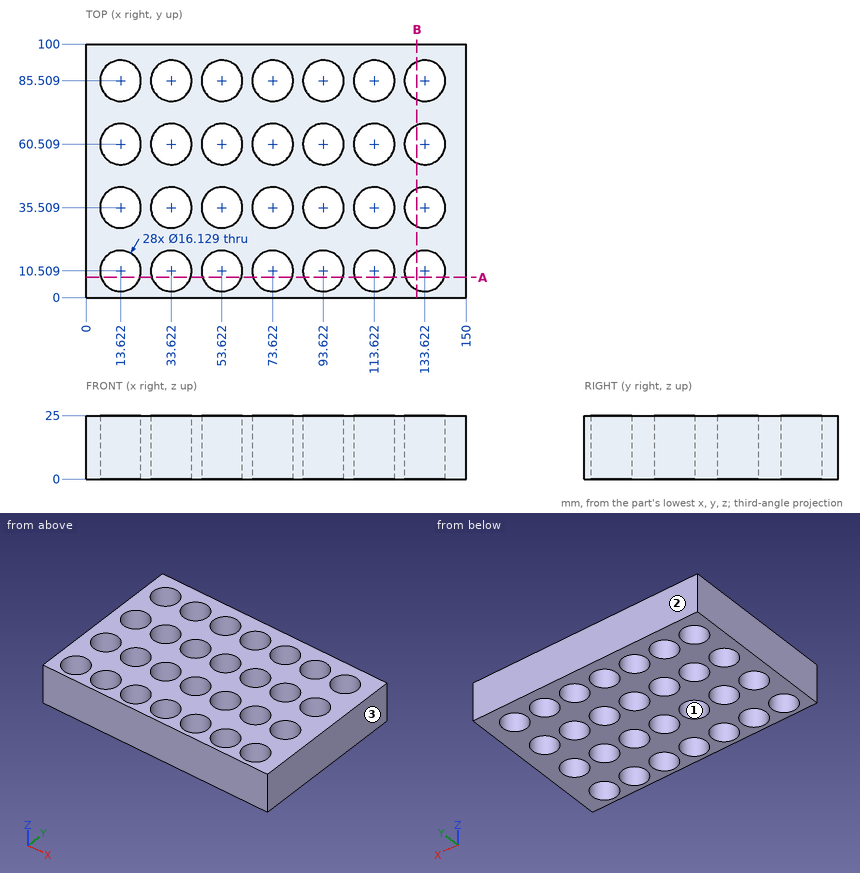
Input: dimensioned drawing with shaded views. Units: mm. Origin: part minimum x, y, z. Give positions to 0.01 mm unless a question says otherwise; leave off trailing zeros. Order: outer loops, then holes, each group sorted by start corner. A loop starts at its lowest first (then second) coordinate and runs counter-clockwise, first axis right, second up. Notation, with made-up numbers: (16.5, 60.25) -> (64.5, 60.25) arc R27 ccw to (64.5, 88.25) -> close; hole circle Ø9 at (-17.75, 82). An arc over 180 degrees is marked (long way). Write item = value, one per line.
Item 1: Ray query, probe 1 along Y at (x, z) = (93, 4); probe 2 along Y at (x, z) = (120.5, 18.25) (1 decimal). Return the intervals inside material, ascending.
Check result:
probe_1 = 0 to 2.47, 18.55 to 27.47, 43.55 to 52.47, 68.55 to 77.47, 93.55 to 100
probe_2 = 0 to 6.3, 14.7 to 31.3, 39.7 to 56.3, 64.7 to 81.3, 89.7 to 100
Item 2: Section query B-B (x = 130.5). Output: boundary loops of the cut face in (y, z) (1 decimal).
Check result:
outline = (0, 0) -> (3.1, 0) -> (3.1, 25) -> (0, 25) -> close; (17.9, 0) -> (28.1, 0) -> (28.1, 25) -> (17.9, 25) -> close; (42.9, 0) -> (53.1, 0) -> (53.1, 25) -> (42.9, 25) -> close; (67.9, 0) -> (78.1, 0) -> (78.1, 25) -> (67.9, 25) -> close; (92.9, 0) -> (100, 0) -> (100, 25) -> (92.9, 25) -> close
Item 3: Mould query, pull axis X, two halves, no side actions, for the marked faces 1, 2 and 3. Classes: +X half, -X half, draft (parallel to the pull), parting line (faces both ways), or undercut.
Check result:
face_1 = undercut
face_2 = draft
face_3 = +X half
Item 4: Contact query for a flat-ended pin moving along its axis: pin 1 (9.5 mm diameter, centred on x = 13.62, y = 10.51, fed in from -Z). Output: stop coordinate, or through.
Check result:
pin_1 = through
Item 5: Section query A-A (y = 8). State how many separate pieces and enclosed holes the cut face has, then the cut area to 3 significant figures.
Check result:
separate_pieces = 8
enclosed_holes = 0
area = 1,070 mm²
